Geometry: final body of the model. Coordinates: model frame, mm. Give positions to 0.01 mm unless a question says otherwise; leave off trailing zeros. Loops run counter-clockwise (first coordinate to the right, second up) from the corner with the lowest first, then second, coordinate; pieces in that order, holes last. Notation, with made-up numbers: (35.25, 17.5) - (91.25, 17.5) arc R32 cw to (91.25, 49.5) - close; hole circle Ø7 at (7, 54). An arc over 180 degrees is marked (long way). Answer in a Markdown table with one row per item.
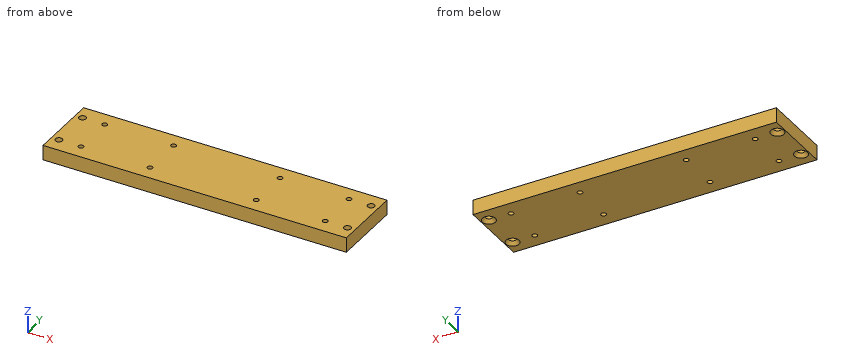
Autodesk Inventor part; units mm, degrees
ref_plane "YZ Plane" through (0, 0, 0) normal (1, 0, 0) x (0, 1, 0)
ref_plane "XZ Plane" through (0, 0, 0) normal (0, 1, 0) x (-1, 0, 0)
ref_plane "XY Plane" through (0, 0, 0) normal (0, 0, 1) x (1, 0, 0)
sketch "Sketch1" plane through (0, 0, 0) normal (0, 0, 1) x (1, 0, 0)
  line L0 (0, 0) -> (195.58, 0)
  line L1 (195.58, 0) -> (195.58, 45.72)
  line L2 (195.58, 45.72) -> (0, 45.72)
  line L3 (0, 45.72) -> (0, 0)
  dimension "d0" = 45.72
  dimension "d1" = 195.58
extrude "Extrusion1" add sketch "Sketch1" along normal blind 9.525
sketch "Sketch2" plane through (0, 0, 0) normal (0, 0, -1) x (-1, 0, 0)
  circle A0 centre (-176.53, 36.195) radius 4.4323
  circle A1 centre (-132.08, 36.195) radius 4.4323
  circle A2 centre (-132.08, 9.525) radius 4.4323
  circle A3 centre (-176.53, 9.525) radius 4.4323
  circle A4 centre (-63.5, 36.195) radius 4.4323
  circle A5 centre (-19.05, 36.195) radius 4.4323
  circle A6 centre (-19.05, 9.525) radius 4.4323
  circle A7 centre (-63.5, 9.525) radius 4.4323
hole "Hole1" at (176.53, 36.195, 0) at (132.08, 36.195, 0) at (132.08, 9.525, 0) at (176.53, 9.525, 0) at (63.5, 9.525, 0) at (63.5, 36.195, 0) at (19.05, 36.195, 0) at (19.05, 9.525, 0) direction (0, 0, 1) diameter 3.302 end through all
sketch "Sketch3" plane through (0, 0, 0) normal (0, 0, -1) x (-1, 0, 0)
  circle A0 centre (-19.05, 9.525) radius 1.651
  circle A1 centre (-19.05, 36.195) radius 1.651
  line L0 (-195.58, 46.9392) -> (-195.58, -0.0508)
  line L1 (-186.055, -0.0508) -> (-195.58, -0.0508)
  line L2 (-186.055, -0.0508) -> (-186.055, 46.9392)
  line L3 (-195.58, 46.9392) -> (-186.055, 46.9392)
  line L4 (0, 46.9392) -> (0, -0.0508)
  line L5 (0, 46.9392) -> (-9.525, 46.9392)
  line L6 (-9.525, -0.0508) -> (-9.525, 46.9392)
  line L7 (-9.525, -0.0508) -> (0, -0.0508)
  circle A2 centre (-4.7625, 36.195) radius 1.651
  circle A3 centre (-4.7625, 9.525) radius 1.651
  line L8 (-195.58, 45.72) -> (0, 45.72)
  point P0 (-4.7625, 9.525)
  point P1 (-4.7625, 36.195)
  point P2 (-190.8175, 36.195)
  point P3 (-190.8175, 9.525)
  dimension "d18" = 9.525
hole "Hole2" at (4.7625, 9.525, 0) at (4.7625, 36.195, 0) at (190.8175, 36.195, 0) at (190.8175, 9.525, 0) direction (0, 0, 1) diameter 4.4958 end through all countersink diameter 8.4328 countersink angle 82
properties part number "MagnetPlate" material "Aluminum-6061"
Q1. Cut plane A-A (x = 132.08). Output: boundary loops of the cut face in (y, z) (3 decimals), and give its area (3 significant figures).
Check values:
| item | result |
|---|---|
| outline | (0, 0) - (7.874, 0) - (7.874, 9.525) - (0, 9.525) - close; (11.176, 0) - (34.544, 0) - (34.544, 9.525) - (11.176, 9.525) - close; (37.846, 0) - (45.72, 0) - (45.72, 9.525) - (37.846, 9.525) - close |
| area | 373 mm² |
Q2. First-contact query: pin 1 (7 mm diameter, centred on x = 4.76, y = 36.2, fed in from +Z) (3 decimals). Flat tip, straight axial feed; report the tip coordinate or a pass-through.
Check values:
| item | result |
|---|---|
| pin 1 | z = 9.525 |
Q3. Material intervals for line 1 along Y through (x, z) = (132.08, 7); line 2 along X through (y, z) = (11.5, 3); line 3 along Y through (x, z) = (176, 8.25), sorted ascending.
Check values:
| item | result |
|---|---|
| line 1 | 0 to 7.87, 11.18 to 34.54, 37.85 to 45.72 |
| line 2 | 0 to 3.69, 5.84 to 189.74, 191.89 to 195.58 |
| line 3 | 0 to 7.96, 11.09 to 34.63, 37.76 to 45.72 |
